from build123d import *

# Parameters (mm, degrees)
F0_R         = 11
F1_DEPTH     = 7
F2_T1_DEPTH  = 44.3442261521
F2_T3_DEPTH  = 44.3442261521
F2_T5_DEPTH  = 44.3442261521
F2_T7_DEPTH  = 44.3442261521
F2_T9_DEPTH  = 44.3442261521
F2_T11_DEPTH = 44.3442261521
F2_T14_ANGLE = 269.2452016921
F2_T16_ANGLE = 269.2452016921
F2_T18_ANGLE = 269.2452016921
F2_T20_ANGLE = 269.2452016921
F2_T22_ANGLE = 269.2452016921
F2_T24_ANGLE = 269.2452016921
F4_DEPTH     = 25.4
F5_DEPTH     = 25.4


# Not quite as in the source:
# - a fillet or chamfer that OpenCascade refuses, or shapes differently, is made with other operations: its cross-section is extruded or revolved along the edge and cut away or added
# - a feature names something its author has since deleted; it is built from what else it names


with BuildPart() as f1:
    # F0 (on Front) → F1 (new body)
    with BuildSketch(Plane.XZ):
        with BuildLine():
            Line((-19.8038627003, 14.4570641122), (-44.8442322709, 0))
            Line((-44.8442322709, 0), (-19.8038627003, -14.4570641122))
            ThreePointArc((-19.8038627003, -14.4570641122), (-8.6430254441, -9.8340939532), (-1.2889419323, -19.4181221799))
            ThreePointArc((-1.2889419323, -19.4181221799), (-1.6270298411, -21.9861548035), (-2.6182534351, -24.3791802476))
            Line((-2.6182534351, -24.3791802476), (22.4221161354, -38.8362443598))
            Line((22.4221161354, -38.8362443598), (22.4221161354, -9.9221161354))
            ThreePointArc((22.4221161354, -9.9221161354), (12.5, 0), (22.4221161354, 9.9221161354))
            Line((22.4221161354, 9.9221161354), (22.4221161354, 38.8362443598))
            Line((22.4221161354, 38.8362443598), (-2.6182534351, 24.3791802476))
            ThreePointArc((-2.6182534351, 24.3791802476), (-1.6270298411, 21.9861548035), (-1.2889419323, 19.4181221799))
            ThreePointArc((-1.2889419323, 19.4181221799), (-8.6430254441, 9.8340939532), (-19.8038627003, 14.4570641122))
        make_face()
        Circle(F0_R, mode=Mode.SUBTRACT)
    extrude(amount=-F1_DEPTH)

    # F2: chamfer of 3 on 18 edges, made by hand

    # F2_s2 → F2_t1 (cut)
    with BuildSketch(Plane(origin=(40.3146025973, 0, 23.2756466618), x_dir=(0, 1, 0), z_dir=(-0.8660254038, 0, -0.5))):
        Polygon((7, -19.4221161354), (4, -22.4221161354), (7, -22.4221161354), align=None)
        Polygon((3, -22.4221161354), (0, -19.4221161354), (0, -22.4221161354), align=None)
    extrude(amount=F2_T1_DEPTH, mode=Mode.SUBTRACT)

    # F2_s4 → F2_t3 (cut)
    with BuildSketch(Plane(origin=(-1.9113762384, 0, -1.1035335858), x_dir=(0, 1, 0), z_dir=(-0.8660254038, 0, -0.5))):
        Polygon((3, -22.4221161354), (0, -19.4221161354), (0, -22.4221161354), align=None)
        Polygon((4, -22.4221161354), (7, -19.4221161354), (7, -22.4221161354), align=None)
    extrude(amount=F2_T3_DEPTH, mode=Mode.SUBTRACT)

    # F2_s6 → F2_t5 (cut)
    with BuildSketch(Plane(origin=(-40.3146025973, 0, 23.2756466618), x_dir=(0, 1, 0), z_dir=(0.8660254038, 0, -0.5))):
        Polygon((0, -19.4221161354), (3, -22.4221161354), (0, -22.4221161354), align=None)
        Polygon((7, -19.4221161354), (4, -22.4221161354), (7, -22.4221161354), align=None)
    extrude(amount=F2_T5_DEPTH, mode=Mode.SUBTRACT)

    # F2_s8 → F2_t7 (cut)
    with BuildSketch(Plane(origin=(1.9113762384, 0, -1.1035335858), x_dir=(0, 1, 0), z_dir=(0.8660254038, 0, -0.5))):
        Polygon((3, -22.4221161354), (0, -19.4221161354), (0, -22.4221161354), align=None)
        Polygon((7, -19.4221161354), (4, -22.4221161354), (7, -22.4221161354), align=None)
    extrude(amount=F2_T7_DEPTH, mode=Mode.SUBTRACT)

    # F2_s10 → F2_t9 (cut)
    with BuildSketch(Plane.XY.offset(-46.5512933237)):
        Polygon((22.4221161354, 3), (19.4221161354, 0), (22.4221161354, 0), align=None)
        Polygon((19.4221161354, 7), (22.4221161354, 4), (22.4221161354, 7), align=None)
    extrude(amount=F2_T9_DEPTH, mode=Mode.SUBTRACT)

    # F2_s12 → F2_t11 (cut)
    with BuildSketch(Plane.XY.offset(2.2070671715)):
        Polygon((22.4221161354, 3), (19.4221161354, 0), (22.4221161354, 0), align=None)
        Polygon((19.4221161354, 7), (22.4221161354, 4), (22.4221161354, 7), align=None)
    extrude(amount=F2_T11_DEPTH, mode=Mode.SUBTRACT)

    # F2_s13 → F2_t14 (revolve, cut)
    with BuildSketch(Plane(origin=(4.0288460704, 0, 15.4420044307), x_dir=(0, 1, 0), z_dir=(0.2524510604, 0, 0.9676096641))):
        Polygon((0, 28.6721698019), (3, 25.6721698019), (0, 25.6721698019), align=None)
    revolve(axis=Axis((-11.2110580677, 0, 19.4181221799), (0, -1, 0)), revolution_arc=F2_T14_ANGLE, mode=Mode.SUBTRACT)

    # F2_s15 → F2_t16 (revolve, cut)
    with BuildSketch(Plane(origin=(-15.3875911575, 0, 4.2319191704), x_dir=(0, 1, 0), z_dir=(-0.9642000803, 0, 0.2651758006))):
        Polygon((7, -28.6721698019), (4, -25.6721698019), (7, -25.6721698019), align=None)
    revolve(axis=Axis((-11.2110580677, 7, 19.4181221799), (0, 1, 0)), revolution_arc=F2_T16_ANGLE, mode=Mode.SUBTRACT)

    # F2_s17 → F2_t18 (revolve, cut)
    with BuildSketch(Plane(origin=(-15.3875911575, 0, -4.2319191704), x_dir=(0, 1, 0), z_dir=(-0.9642000803, 0, -0.2651758006))):
        Polygon((3, 25.6721698019), (0, 28.6721698019), (0, 25.6721698019), align=None)
    revolve(axis=Axis((-11.2110580677, 0, -19.4181221799), (0, -1, 0)), revolution_arc=F2_T18_ANGLE, mode=Mode.SUBTRACT)

    # F2_s19 → F2_t20 (revolve, cut)
    with BuildSketch(Plane(origin=(4.0288460704, 0, -15.4420044307), x_dir=(0, 1, 0), z_dir=(0.2524510604, 0, -0.9676096641))):
        Polygon((7, -28.6721698019), (4, -25.6721698019), (7, -25.6721698019), align=None)
    revolve(axis=Axis((-11.2110580677, 7, -19.4181221799), (0, 1, 0)), revolution_arc=F2_T20_ANGLE, mode=Mode.SUBTRACT)

    # F2_s21 → F2_t22 (revolve, cut)
    with BuildSketch(Plane(origin=(11.3587450871, 0, 11.2100852602), x_dir=(0, 1, 0), z_dir=(0.7117490199, 0, 0.7024338636))):
        Polygon((3, -25.6721698019), (0, -28.6721698019), (0, -25.6721698019), align=None)
    revolve(axis=Axis((22.4221161354, 0, 0), (0, 1, 0)), revolution_arc=F2_T22_ANGLE, mode=Mode.SUBTRACT)

    # F2_s23 → F2_t24 (revolve, cut)
    with BuildSketch(Plane(origin=(11.3587450871, 0, 11.2100852602), x_dir=(0, 1, 0), z_dir=(0.7117490199, 0, 0.7024338636))):
        Polygon((7, -28.6721698019), (4, -25.6721698019), (7, -25.6721698019), align=None)
    revolve(axis=Axis((22.4221161354, 7, 0), (0, 1, 0)), revolution_arc=F2_T24_ANGLE, mode=Mode.SUBTRACT)

    # F3 (on face) → F4 (cut)
    with BuildSketch(Plane.XZ):
        Polygon((13.0480463402, 22.5998792008), (6.3740697952, 11.0402127363), (6.4247100072, 10.9550491246), (13.1471202974, 11.0414866405), (16.4334683579, 16.9064834844), align=None)
        Polygon((2.9886477775, 16.7336084526), (6.3740697952, 11.0402127363), (13.0480463402, 22.5998792008), (12.9974061282, 22.6850428125), (6.274995838, 22.5986052966), align=None)
        Polygon((-26.1366, 0), (-12.7, 0), (-16.05915, 5.8182184702), (-22.77745, 5.8182184702), align=None)
        Polygon((-16.05915, -5.8182184702), (-12.7, 0), (-26.1366, 0), (-22.77745, -5.8182184702), align=None)
    extrude(amount=-F4_DEPTH, mode=Mode.SUBTRACT)

    # F3 (on face) → F5 (cut)
    with BuildSketch(Plane.XZ):
        Polygon((2.9886477775, 16.7336084526), (6.3740697952, 11.0402127363), (13.0480463402, 22.5998792008), (12.9974061282, 22.6850428125), (6.274995838, 22.5986052966), align=None)
        Polygon((13.0480463402, 22.5998792008), (6.3740697952, 11.0402127363), (6.4247100072, 10.9550491246), (13.1471202974, 11.0414866405), (16.4334683579, 16.9064834844), align=None)
        Polygon((-16.05915, -5.8182184702), (-12.7, 0), (-26.1366, 0), (-22.77745, -5.8182184702), align=None)
        Polygon((-26.1366, 0), (-12.7, 0), (-16.05915, 5.8182184702), (-22.77745, 5.8182184702), align=None)
        Polygon((13.0581752927, -11.0105414452), (6.3398781361, -11.0043602821), (13.0474692042, -22.6469734606), (16.4119708267, -16.8318480344), align=None)
        Polygon((13.0474692042, -22.6469734606), (6.3398781361, -11.0043602821), (2.9753765137, -16.8194857083), (6.3291720477, -22.6407922976), align=None)
    extrude(amount=-F5_DEPTH, mode=Mode.SUBTRACT)


solid = f1.part
Check sheet for the modelled part. Datum: model origin and axes. Units: mm. A direction names the side the tool comes from. Round coordinates to 2 decimals unless told otherwise and drop trailing zeros. Loops run counter-clockwise (first coordinate to the right, second up) from the corner with the lowest first, then second, coordinate; pieces in that order, holes last.
1. Scan lines: probe 1 along Z at (x, y) = (14, 1.5); probe 2 along Z at (x, y) = (0, 2); probe 3 along Z at (x, y) = (-20.5, 1.75). Record each from-to range of solid material in increasing order.
2. Set-up check for faces 5 (the flat face through (-32.15, 3.49, 7.33)), 6 (the flat face through (4.68, 3.45, -13.87)): record each of +Z, -Z, +X, -X, +Y, -Y from which the full face is reachable in a straight line by a thin tool's end or side.
3. Mould release check, pull along X, two halves, no side actions. Record for faces 1 (the flat face through (-24.434, 3.451, 2.95)), 2 (the flat face through (9.73, 3.49, -31.51)), 3 (the conical face through (-6.37, 4.146, -10.591)), 4 (the flat face through (20.9, 5.52, 24.18)): released by +X, released by -X, zero draft, split by the parting line, or undercut.
4. Sectioned sample at C-C on z = 32.5. Record the boundary of the cut face in (x, y).
5. Sectioned sample at A-A on x = -25. Record the boundary of the cut face in (y, z), and give its area (3 significant figures).
6. Sectioned sample at B-B on x = 5. Record the boundary of the cut face in (y, z), and give its area (3 significant figures).
7. Gauge pin test, flat ends, axial feed: pin 1 Ø6 at (x, z) = (-1.5, -20.5) entering from -Y; pin 2 Ø3.5 at (x, y) = (-19.5, 3) entering from -Z; pin 3 Ø1 at (y, z) = (5.5, -30) entering from +X. Record the tip position at first contact, or that the pin passes through.
Recorded:
1. probe 1: z = -32.24 to -21, -12.65 to -7.72, 7.72 to 12.56, 21 to 32.24
1. probe 2: z = -24.74 to -11, 11 to 24.74
1. probe 3: z = -12.61 to -5.82, 5.82 to 12.61
2. face 5: +Z, -X, +Y, -Y
2. face 6: +Y, -Y
3. face 1: undercut
3. face 2: released by -X
3. face 3: undercut
3. face 4: released by +X
4. outline: (11.45, 3) - (17.45, 0) - (19.42, 0) - (22.42, 3) - (22.42, 4) - (19.42, 7) - (17.45, 7) - (11.45, 4) - close
5. outline: (0, -7.99) - (3, -11.46) - (4, -11.46) - (7, -7.99) - (7, -1.97) - (0, -1.97) - close; (0, 1.97) - (7, 1.97) - (7, 7.99) - (4, 11.46) - (3, 11.46) - (0, 7.99) - close
5. area: 112 mm2
6. outline: (0, -25.31) - (3, -28.78) - (4, -28.78) - (7, -25.31) - (7, -20.33) - (0, -20.33) - close; (0, -13.32) - (7, -13.32) - (7, -9.8) - (0, -9.8) - close; (0, 9.8) - (7, 9.8) - (7, 13.35) - (0, 13.35) - close; (0, 20.32) - (7, 20.32) - (7, 25.31) - (4, 28.78) - (3, 28.78) - (0, 25.31) - close
6. area: 147 mm2
7. pin 1: stops at y = 0.15
7. pin 2: stops at z = -14.46
7. pin 3: stops at x = 21.42
